Part model, mm, in its own coordinate system. Round coordinates to 2 decimals unless told otherwise and drop trailing zeros. Write each loop counter-clockwise with the first axis right and the second up, starting at its lowest first coordinate (ties: lowest second). Pieces come first, ordered by that corner, then holes.
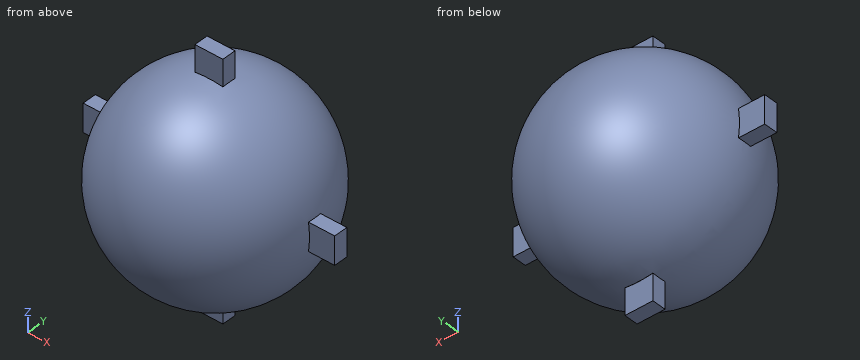
```python
from build123d import *

# Parameters (mm, degrees)
SHELL1_T                 = 3.175
BOSS_EXTRUDE1_REACH      = 730.747
BOSS_EXTRUDE1_END_RADIUS = 274.32
SKETCH4_W                = 76.2
SKETCH4_H                = 38.1
CIRPATTERN1_COUNT        = 4


with BuildPart() as part:
    # Sketch1 → Revolve6 (revolve)
    with BuildSketch(Plane(origin=(0, 0, 0), x_dir=(1, 0, 0), z_dir=(0, 1, 0))):
        with BuildLine():
            Line((-274.32, 0), (274.32, 0))
            ThreePointArc((274.32, 0), (0, 274.32), (-274.32, 0))
        make_face()
    revolve(axis=Axis((-274.32, 0, 0), (1, 0, 0)))

    # Shell1 (no face opened: a closed hollow body)
    add(offset(amount=-SHELL1_T, mode=Mode.PRIVATE), mode=Mode.SUBTRACT)

    # Boss-Extrude1: up to this sphere (the profile starts outside it)
    boss_extrude1_end = Location((0, 0, 0)) * Sphere(BOSS_EXTRUDE1_END_RADIUS, mode=Mode.PRIVATE)
    # Sketch4 → Boss-Extrude1 (add, up to the surface)
    with BuildSketch(Plane.XY.offset(342.5825), mode=Mode.PRIVATE) as boss_extrude1_sk1:
        Rectangle(SKETCH4_W, SKETCH4_H)
    boss_extrude1_tool1 = extrude(boss_extrude1_sk1.sketch, amount=-BOSS_EXTRUDE1_REACH, mode=Mode.PRIVATE) - boss_extrude1_end
    boss_extrude1 = boss_extrude1_tool1.solids().sort_by_distance((0, 0, 342.5825))[0]
    add(boss_extrude1)

    # CirPattern1: Boss-Extrude1 ×4 about axis
    cirpattern1_axis = Axis((0, 0, 0), (0, 1, 0))
    for i in range(1, CIRPATTERN1_COUNT):
        add(boss_extrude1.rotate(cirpattern1_axis, i * 360 / CIRPATTERN1_COUNT))


solid = part.part
```
Q1. Cut at C-C on y = -185. Write the cut outline in (x, z), plus the area to 3 significant figures.
Values follow:
outline: circle Ø405.1 at (0, 0); hole circle Ø396.46 at (0, 0)
area: 5,440 mm2
Q2. Cut at A-A on z = -15. Write the cut outline in (x, y), plus the area to 3 significant figures.
Values follow:
outline: (-342.58, -19.05) - (-273.25, -19.05) arc R273.91 ccw to (273.25, -19.05) - (342.58, -19.05) - (342.58, 19.05) - (273.25, 19.05) arc R273.91 ccw to (-273.25, 19.05) - (-342.58, 19.05) - close; hole circle Ø541.46 at (0, 0)
area: 10,700 mm2
Q3. Drop flat-ended pins along their axis: pin 1 (11.5 mm diameter, centred on x = -314, y = -3, fed in from +Z); pin 2 (21.5 mm diameter, centred on x = 0.5, z = 304, fed in from +Y); pin 3 (12 mm diameter, centred on x = -205.5, z = 132.5, fed in from -Y). Give the stop position or say it passes through.
Values follow:
pin 1: stops at z = 38.1
pin 2: stops at y = 19.05
pin 3: stops at y = -135.51
Q4. Wall check: L1, parallel to X at y = 35.5, z = -55.5; L2, parallel to Y at x = 80, z = -23.5; L3, parallel to Z at x = -9.5, y = -68. Give the ranges that are in metal, low to high.
Values follow:
L1: x = -266.29 to -263.02, 263.02 to 266.29
L2: y = -261.34 to -258.01, 258.01 to 261.34
L3: z = -265.59 to -262.31, 262.31 to 265.59
